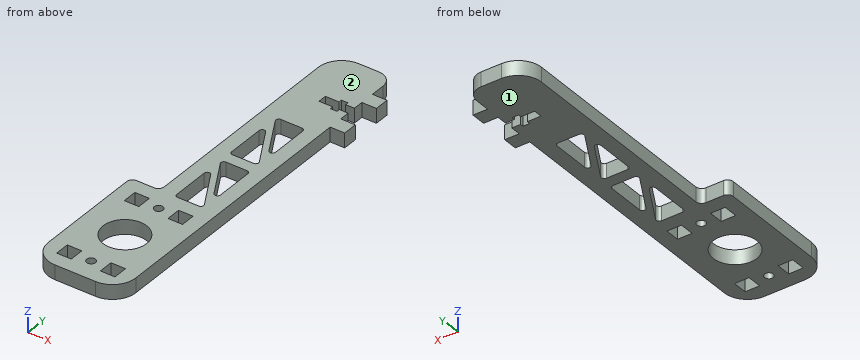
from build123d import *

# Parameters (mm, degrees)
ESQUISSE1_R        = 7.5
ESQUISSE1_R_2      = 1.5
ESQUISSE1_W        = 5
ESQUISSE1_H        = 5
BOSS_EXTRU_1_DEPTH = 5


with BuildPart() as part:
    # Esquisse1 → Boss.-Extru.1 (new body)
    with BuildSketch(Plane.XY):
        with BuildLine():
            Line((0, 0), (0, -92))
            ThreePointArc((0, -92), (-2.343145751, -97.656854249), (-8, -100))
            Line((-8, -100), (-22, -100))
            ThreePointArc((-22, -100), (-27.656854249, -97.656854249), (-30, -92))
            Line((-30, -92), (-30, -55))
            ThreePointArc((-30, -55), (-29.414213562, -53.585786438), (-28, -53))
            Line((-28, -53), (-22, -53))
            ThreePointArc((-22, -53), (-20.585786438, -52.414213562), (-20, -51))
            Line((-20, -51), (-20, 22))
            ThreePointArc((-20, 22), (-17.656854249, 27.656854249), (-12, 30))
            Line((-12, 30), (-5, 30))
            ThreePointArc((-5, 30), (-1.464466094, 28.535533906), (0, 25))
            Line((0, 25), (0, 20))
            Line((0, 20), (5, 20))
            Line((5, 20), (5, 15))
            Line((5, 15), (0, 15))
            Line((0, 15), (0, 11.5))
            Line((0, 11.5), (-3, 11.5))
            Line((-3, 11.5), (-3, 12.6))
            Line((-3, 12.6), (-5.3, 12.6))
            Line((-5.3, 12.6), (-5.3, 11.5))
            Line((-5.3, 11.5), (-10, 11.5))
            Line((-10, 11.5), (-10, 8.5))
            Line((-10, 8.5), (-5.3, 8.5))
            Line((-5.3, 8.5), (-5.3, 7.4))
            Line((-5.3, 7.4), (-3, 7.4))
            Line((-3, 7.4), (-3, 8.5))
            Line((-3, 8.5), (0, 8.5))
            Line((0, 8.5), (0, 5))
            Line((0, 5), (5, 5))
            Line((5, 5), (5, 0))
            Line((5, 0), (0, 0))
        make_face()
        with Locations((-15, -76.5)):
            Circle(ESQUISSE1_R, mode=Mode.SUBTRACT)
        with Locations((-15, -60.5)):
            Circle(ESQUISSE1_R_2, mode=Mode.SUBTRACT)
        with Locations((-15, -92.5)):
            Circle(ESQUISSE1_R_2, mode=Mode.SUBTRACT)
        with Locations((-7.5, -92.5)):
            Rectangle(ESQUISSE1_W, ESQUISSE1_H, mode=Mode.SUBTRACT)
        with Locations((-22.5, -92.5)):
            Rectangle(ESQUISSE1_W, ESQUISSE1_H, mode=Mode.SUBTRACT)
        with Locations((-22.5, -60.5)):
            Rectangle(ESQUISSE1_W, ESQUISSE1_H, mode=Mode.SUBTRACT)
        with Locations((-7.5, -60.5)):
            Rectangle(ESQUISSE1_W, ESQUISSE1_H, mode=Mode.SUBTRACT)
        with BuildLine():
            Line((-6, -5), (-13.295840542, -5))
            ThreePointArc((-13.295840542, -5), (-14.158315423, -5.493900129), (-14.168837394, -6.487725842))
            Line((-14.168837394, -6.487725842), (-6.872996852, -19.546795671))
            ThreePointArc((-6.872996852, -19.546795671), (-5.748004813, -20.026798317), (-5, -19.059069829))
            Line((-5, -19.059069829), (-5, -6))
            ThreePointArc((-5, -6), (-5.292893219, -5.292893219), (-6, -5))
        make_face(mode=Mode.SUBTRACT)
        with BuildLine():
            Line((-13.127003148, -12.453204329), (-5.831162606, -25.512274158))
            ThreePointArc((-5.831162606, -25.512274158), (-5.841684577, -26.506099871), (-6.704159458, -27))
            Line((-6.704159458, -27), (-14, -27))
            ThreePointArc((-14, -27), (-14.707106781, -26.707106781), (-15, -26))
            Line((-15, -26), (-15, -12.940930171))
            ThreePointArc((-15, -12.940930171), (-14.251995187, -11.973201683), (-13.127003148, -12.453204329))
        make_face(mode=Mode.SUBTRACT)
        with BuildLine():
            Line((-6, -31), (-13.295840542, -31))
            ThreePointArc((-13.295840542, -31), (-14.158315423, -31.493900129), (-14.168837394, -32.487725842))
            Line((-14.168837394, -32.487725842), (-6.872996852, -45.546795671))
            ThreePointArc((-6.872996852, -45.546795671), (-5.748004813, -46.026798317), (-5, -45.059069829))
            Line((-5, -45.059069829), (-5, -32))
            ThreePointArc((-5, -32), (-5.292893219, -31.292893219), (-6, -31))
        make_face(mode=Mode.SUBTRACT)
        with BuildLine():
            Line((-13.127003148, -38.453204329), (-5.831162606, -51.512274158))
            ThreePointArc((-5.831162606, -51.512274158), (-5.841684577, -52.506099871), (-6.704159458, -53))
            Line((-6.704159458, -53), (-14, -53))
            ThreePointArc((-14, -53), (-14.707106781, -52.707106781), (-15, -52))
            Line((-15, -52), (-15, -38.940930171))
            ThreePointArc((-15, -38.940930171), (-14.251995187, -37.973201683), (-13.127003148, -38.453204329))
        make_face(mode=Mode.SUBTRACT)
    extrude(amount=BOSS_EXTRU_1_DEPTH)


solid = part.part
CAD build for the part. Positions are in the model's coordinates, mm. Face numbers are marked on the shaded views. Coordinates: 2 decimals unless noted, no trailing zeros. Loops run counter-clockwise (first coordinate to the right, second up) from the corner with the lowest first, then second, coordinate; pieces in that order, holes last. Notation, with made-up numbers: (51, -27.75) - (109, -27.75) arc R14 cw to (109, -15.75) - close; hole circle Ø6 at (-39.75, 82.25). An arc over 180 degrees is marked (long way). Write item = value, one per line. Start each with the question number.
Q1. Flat gauge pins, fed straight in: pin 1 Ø0.7 at (x, z) = (-4.5, 1.5) entering from -Y; pin 2 Ø0.5 at (y, z) = (12, 3) entering from +X; pin 3 Ø0.7 at (x, z) = (-4.5, 2.5) entering from +Y. Where does each tip first touch, or does it go through?
Q2. Pull direction Z, two halves, no side cores. Call the marked faces 1 and 2: pulls with the +Z half, pulls with the -Z half, needs draft (parallel to the pull), parting line crosses it, or undercut.
Q3. Drill centre lines: L1, parallel to X at y = -92.5, z = 3.35; L2, parallel to Y at x = -23, z = 3.85; L3, parallel to X at y = -89, z = 0.5. Where is each one in solid material? Low to high.
Q4. Cut at B-B, the plane x = 2. List the corners of the cut face in (y, z), then the cut area to 3 significant figures.
Q5. Cut at C-C, the plane y = -60.5. List the corners of the cut face in (x, z).
Q6. Cut at D-D, the plane z = 3.85. Give the number of separate pieces and of enclosed holes in the cut face, then the cut area to 3 significant figures.
Q7. Cut at A-A, the plane y = -76.5. List the corners of the cut face in (x, z), then the cut area to 3 significant figures.
Computed:
q1.pin_1 = -99.35
q1.pin_2 = 0
q1.pin_3 = 30
q2.face_1 = pulls with the -Z half
q2.face_2 = pulls with the +Z half
q3.L1 = -29.98 to -25, -20 to -16.5, -13.5 to -10, -5 to -0.02
q3.L2 = -99.94 to -95, -90 to -63, -58 to -53
q3.L3 = -30 to 0
q4.outline = (0, 0) - (5, 0) - (5, 5) - (0, 5) - close; (15, 0) - (20, 0) - (20, 5) - (15, 5) - close
q4.area = 50.0 mm²
q5.outline = (-30, 0) - (-25, 0) - (-25, 5) - (-30, 5) - close; (-20, 0) - (-16.5, 0) - (-16.5, 5) - (-20, 5) - close; (-13.5, 0) - (-10, 0) - (-10, 5) - (-13.5, 5) - close; (-5, 0) - (0, 0) - (0, 5) - (-5, 5) - close
q6.separate_pieces = 1
q6.enclosed_holes = 11
q6.area = 2,400 mm²
q7.outline = (-30, 0) - (-22.5, 0) - (-22.5, 5) - (-30, 5) - close; (-7.5, 0) - (0, 0) - (0, 5) - (-7.5, 5) - close
q7.area = 75.0 mm²
